Check sheet for the modelled part. Datum: model origin and axes. Units: mm. Face numbers are marked on the shaded views. A direction names the side the tool comes from. Round coordinates to 2 decimals unless told otherwise and drop trailing zeros. Order: outer loops, then holes, each group sorted by start corner. A loop starts at its lowest first (then second) coordinate and runs counter-clockwise, first axis right, second up. Notation, with made-up numbers: (-36.5, 47) -> (-23.5, 47) arc R17 cw to (-23.5, 59) -> close; hole circle Ø3 at (55, 70.5). An arc over 180 degrees is marked (long way). Use CSV: the item, a comma, the result in double quotes.
Autodesk Fusion 360 part; units mm, degrees
sketch "Sketch5" plane through (0, 0, 0) normal (0, 0, 1) x (1, 0, 0)
  line L0 (1.15, 4.15) -> (-1.15, 4.15)
  line L1 (-1.15, -4.15) -> (1.15, -4.15)
  line L2 (1.15, -4.15) -> (1.15, 4.15)
  line L3 (1.15, 4.15) -> (-1.15, -4.15) construction
  line L4 (-1.15, 4.15) -> (1.15, -4.15) construction
  line L5 (-4.1, 0.9) -> (-4.1, -0.9)
  line L6 (-4.1, -0.9) -> (-1.15, -0.9)
  line L7 (1.15, -0.9) -> (1.15, 0.9)
  line L8 (-1.15, 0.9) -> (-4.1, 0.9)
  line L9 (-1.15, 4.15) -> (-1.15, 0.9)
  line L10 (-1.15, -0.9) -> (-1.15, -4.15)
  dimension "d16" = 2.3
  dimension "d17" = 8.3
  dimension "d18" = 1.8
  dimension "d20" = 2.95
extrude "Extrude4" add sketch "Sketch5" along normal blind 9.892
equation "d16 = 2.5 mm - 0.2 mm"
equation "d17 = 8.60 mm - 0.3 mm"
equation "d18 = 2 mm - 0.2 mm"
equation "d20 = 3.05 mm - 0.1 mm"
equation "d21 = 8.092 mm - 0.2 mm + 2 mm"
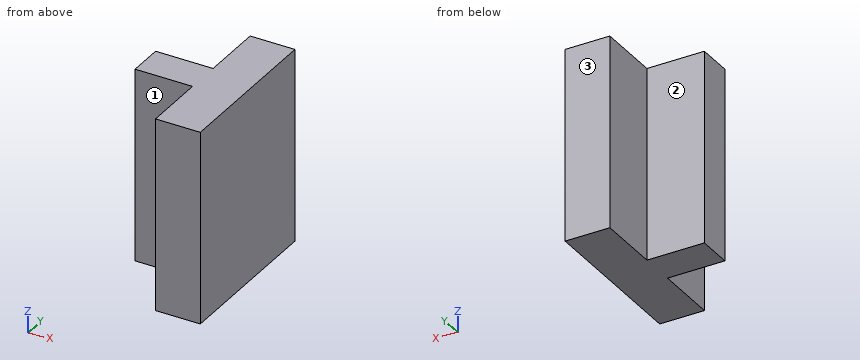
Q1. Sectioned sample at B-B, the plane x = -2.65. Enter the section's corners in (y, z).
Result sheet:
outline,"(-0.9, 0) -> (0.9, 0) -> (0.9, 9.89) -> (-0.9, 9.89) -> close"
Q2. Go/stop test with flat-tipped pins: pin 1 (2.5 mm diameter, centred on x = -3, z = 3.5, fed in from +Y); pin 2 (2.5 mm diameter, centred on x = -3.5, z = 2.5, fed in from -Y); pin 3 (2.5 mm diameter, centred on y = 2.5, z = 3, fed in from -X). Record where each tip stops, or that it passes through.
Result sheet:
pin 1,"stops at y = 0.9"
pin 2,"stops at y = -0.9"
pin 3,"stops at x = -1.15"
Q3. Sectioned sample at C-C, the plane y = -3.5. Enter the section's corners in (x, z).
Result sheet:
outline,"(-1.15, 0) -> (1.15, 0) -> (1.15, 9.89) -> (-1.15, 9.89) -> close"
Q4. Access from +Z, -Z, +X, -X, +Y, -Y to the whole of each face (thin tool, end or side, straight path). Record for the marked faces 1, 2 and 3.
Result sheet:
face 1,"+Z, -Z, -X, -Y"
face 2,"+Z, -Z, -X, +Y"
face 3,"+Z, -Z, +X, -X, +Y"
Q5. Sectioned sample at A-A, the plane z = 2.5. Enter the section's corners in (x, y), then the cut area to 3 significant figures.
Result sheet:
outline,"(-4.1, -0.9) -> (-1.15, -0.9) -> (-1.15, -4.15) -> (1.15, -4.15) -> (1.15, 4.15) -> (-1.15, 4.15) -> (-1.15, 0.9) -> (-4.1, 0.9) -> close"
area,"24.4 mm^2"
Q6. Scan lines: L1, parallel to X at y = 2.5, z = 3.75; L2, parallel to Y at x = -2.9, z = 6.25. Record each from-to range of solid material in increasing order.
Result sheet:
L1,"x = -1.15 to 1.15"
L2,"y = -0.9 to 0.9"
